from build123d import *

# Parameters (mm, degrees)
BOSS_EXTRUDE1_DEPTH    = 30
SKETCH2_W              = 35
SKETCH2_H              = 20
BOSS_EXTRUDE2_DEPTH    = 300
F_10_0MM_DOWEL_HOLE1_D = 10


with BuildPart() as part:
    # Sketch1 → Boss-Extrude1 (new body)
    with BuildSketch(Plane(origin=(0, 0, 0), x_dir=(1, 0, 0), z_dir=(0, 1, 0))):
        with BuildLine():
            Line((0, 35), (0, 0))
            Line((0, 0), (59.446550687, 0))
            ThreePointArc((59.446550687, 0), (290.555085126, 17.296607549), (517.979369235, 61.889458105))
            ThreePointArc((517.979369235, 61.889458105), (560.727418369, 77.204818483), (600, 100))
            ThreePointArc((600, 100), (302.095278427, 48.158968364), (0, 35))
        make_face()
    extrude(amount=BOSS_EXTRUDE1_DEPTH)

    # Sketch2 → Boss-Extrude2 (add)
    with BuildSketch(Plane.ZY):
        with Locations((-17.5, 15)):
            Rectangle(SKETCH2_W, SKETCH2_H)
    extrude(amount=BOSS_EXTRUDE2_DEPTH)

    # Ø10.0mm Dowel Hole1 (through all)
    with Locations(Plane(origin=(0, 25, 0), x_dir=(1, 0, 0), z_dir=(0, 1, 0))):
        with Locations((-200, 17.5), (-100, 17.5)):
            Hole(F_10_0MM_DOWEL_HOLE1_D / 2)


solid = part.part
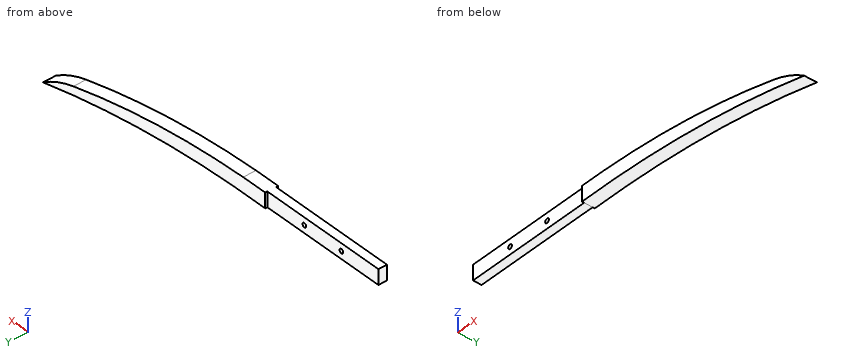
The listing builds one solid part. Answer for the finished solid, in the listing's coordinates (mm). Coordinates: 2 decimals unless noted, no trailing zeros. Write each loop counter-clockwise with the first axis right and the second up, starting at its lowest first coordinate (ties: lowest second). Pieces come first, ordered by that corner, then holes. Notation, with made-up numbers: (37.25, 7.5) -> (83.25, 7.5) arc R24 ccw to (83.25, 37.5) -> close; hole circle Ø8 at (-10, 48). An arc over 180 degrees is marked (long way). One line per question, with ' | ' between items.
1. Straight lines are drawn through the part: line 1 (Z direction, x = -200, y = 18.5); line 2 (Y direction, x = -125.5, z = -15); line 3 (Z direction, x = -138, y = 17.5). For each, find the intervals that lie inside material, in ascending order.
Verdict:
line 1: z = -35 to -22.5, -12.5 to 0 | line 2: y = 5 to 25 | line 3: z = -35 to 0
2. Section B-B (x = -232) is taken. Determine the outline of the cut face in (y, z), and give its area (3 significant figures).
Verdict:
outline: (5, -35) -> (25, -35) -> (25, 0) -> (5, 0) -> close | area: 700 mm^2
3. Section A-A (y = 10.5) is taken. Determine the outline of the cut face in (x, z), and give its area (3 significant figures).
Verdict:
outline: (-300, -35) -> (0, -35) arc R2350 cw to (600, -100) arc R250 ccw to (517.98, -61.89) arc R1950 ccw to (59.45, 0) -> (-300, 0) -> close; hole circle Ø10 at (-200, -17.5); hole circle Ø10 at (-100, -17.5) | area: 26,700 mm^2
4. Given pin 1 Ø1 at (y, z) = (13, -87.5) entering from +X; pin 2 Ø4 at (y, z) = (2, -9.5) entering from -X; pin 3 Ø16 at (x, y) = (-154.5, 18) entering from -Z, each flat-ended and moving along its own axis, determine where each tip first touches the part or whether it passes through.
Verdict:
pin 1: stops at x = 581.38 | pin 2: stops at x = 0 | pin 3: stops at z = -35
